from build123d import *

# Parameters (mm, degrees)
SKETCH1_W           = 5
SKETCH1_H           = 30
SKETCH1_R           = 1
BOSS_EXTRUDE1_DEPTH = 1
FILLET5_R           = 2
FILLET6_R           = 2
FILLET7_R           = 2
FILLET8_R           = 2


with BuildPart() as part:
    # Sketch1 → Boss-Extrude1 (new body)
    with BuildSketch(Plane.XY):
        with Locations((2.5, 15)):
            Rectangle(SKETCH1_W, SKETCH1_H)
        with Locations((2.5, 2.5)):
            Circle(SKETCH1_R, mode=Mode.SUBTRACT)
        with Locations((2.5, 27.5)):
            Circle(SKETCH1_R, mode=Mode.SUBTRACT)
    extrude(amount=BOSS_EXTRUDE1_DEPTH)

    # Fillet5
    fillet5_edges = [part.edges().sort_by_distance(p)[0] for p in [
        (5, 0, 0.5),
    ]]
    fillet(fillet5_edges, radius=FILLET5_R)

    # Fillet6
    fillet6_edges = [part.edges().sort_by_distance(p)[0] for p in [
        (0, 0, 0.5),
    ]]
    fillet(fillet6_edges, radius=FILLET6_R)

    # Fillet7
    fillet7_edges = [part.edges().sort_by_distance(p)[0] for p in [
        (0, 30, 0.5),
    ]]
    fillet(fillet7_edges, radius=FILLET7_R)

    # Fillet8
    fillet8_edges = [part.edges().sort_by_distance(p)[0] for p in [
        (5, 30, 0.5),
    ]]
    fillet(fillet8_edges, radius=FILLET8_R)


solid = part.part
The listing builds one solid part. Answer for the finished solid, in the listing's coordinates (mm). Give positions to 0.01 mm unless a question says otherwise; leave off trailing zeros. Write each loop counter-clockwise with the first axis right and the second up, starting at its lowest first coordinate (ties: lowest second). Pieces come first, ordered by that corner, then holes.
1) Section A-A (y = 2.5) is taken. Write down the section's boundary in (x, z).
2) Section C-C (z = 0.6) is taken. Write down the section's boundary in (x, y), and give its area (3 significant figures).
3) Find the intervals of material crossed by L1, parallel to Y at x = 2.5, z = 0.8; L2, parallel to Y at x = 1.9, z = 0.95; L3, parallel to X at y = 1.75, z = 0.9, in increasing order.
4) Section B-B (x = 2.5) is taken. Write down the section's boundary in (y, z).
5) For a pull along X with two mould halves and no side action, classify faces 1 (the face through (2, 15, 1)), 2 (the face through (1.5, 2.5, 0.5)), 3 (the face through (0, 14.8, 0.5)) as pulls with the +X half, pulls with the -X half, needs draft (parallel to the pull), parting line crosses it, or undercut.
Response:
1. outline: (0, 0) - (1.5, 0) - (1.5, 1) - (0, 1) - close; (3.5, 0) - (5, 0) - (5, 1) - (3.5, 1) - close
2. outline: (0, 2) arc R2 ccw to (2, 0) - (3, 0) arc R2 ccw to (5, 2) - (5, 28) arc R2 ccw to (3, 30) - (2, 30) arc R2 ccw to (0, 28) - close; hole circle Ø2 at (2.5, 2.5); hole circle Ø2 at (2.5, 27.5)
2. area: 140 mm2
3. L1: y = 0 to 1.5, 3.5 to 26.5, 28.5 to 30
3. L2: y = 0 to 1.7, 3.3 to 26.7, 28.3 to 30
3. L3: x = 0.02 to 1.84, 3.16 to 4.98
4. outline: (0, 0) - (1.5, 0) - (1.5, 1) - (0, 1) - close; (3.5, 0) - (26.5, 0) - (26.5, 1) - (3.5, 1) - close; (28.5, 0) - (30, 0) - (30, 1) - (28.5, 1) - close
5. face 1: needs draft
5. face 2: undercut
5. face 3: pulls with the -X half
